Source: CAD feature listing. Evaluate the final solid. Frame: model axes, mm. Face numbers are marked on the shaded views. A direction names the side the tool comes from. Round coordinates to 2 decimals unless told otherwise and drop trailing zeros. Loops run counter-clockwise (first coordinate to the right, second up) from the corner with the lowest first, then second, coordinate; pieces in that order, holes last.
Item 1: Access query for the marked faces 5, 6, 7, 8 and 9. Directions: +Z, -Z, +X, -X, +Y, -Y. A direction counts if a zero-diameter tool reaches every point of the face in a straight line with its end or side. Return the directions, or none.
Item 2: Section query B-B on x = -0.25. Return loops of the section in (y, z), then the cut area to 3 significant figures.
Item 3: Section query A-A on z = 0.4. Return loops of the section in (x, y), then the cut area to 3 significant figures.
Item 4: Pull-direction query (X, two-part tool) for the marked faces 1, 2, 3 and 4; classes: released by +X, released by -X, zero draft, split by the parting line, or undercut.
Item 5: Section query D-D on y = -2.55. Return loops of the section in (x, z).
Item 6: First-contact query: P1, Ø0.8, axis at y = -2.5, z = 1, coming from the -X side; P2, Ø1.1, axis at y = 2.5, z = 1.5, coming from the +X side; P3, Ø3, axis at x = -2, z = 3.5, coming from the -Y side. Flat tips, straight axial feed; report the tip coordinate or a pass-through.
Item 7: Ray query, L1, parallel to Y at x = -3, z = 3.45; L2, parallel to Y at x = -0.5, z = 1.05; L3, parallel to Y at x = 1.75, z = 2.2. Return the intervals inside material, ascending.
Item 8: Section query C-C on x = 1.25. Return loops of the section in (y, z).
```python
from build123d import *

# Parameters (mm, degrees)
BOSS_EXTRUDE1_DEPTH = 6
CUT_EXTRUDE1_DEPTH  = 2
CUT_EXTRUDE2_DEPTH  = 2
CUT_EXTRUDE3_DEPTH  = 2
CUT_EXTRUDE4_DEPTH  = 3


with BuildPart() as part:
    # Sketch1 → Boss-Extrude1 (new body)
    with BuildSketch(Plane.XY):
        with BuildLine():
            Line((0, 2), (-4, 2))
            Line((-4, 2), (-4, 3))
            Line((-4, 3), (0, 3))
            ThreePointArc((0, 3), (3, 0), (0, -3))
            Line((0, -3), (-1, -3))
            Line((-1, -3), (-1, -2))
            Line((-1, -2), (0, -2))
            ThreePointArc((0, -2), (2, 0), (0, 2))
        make_face()
    extrude(amount=BOSS_EXTRUDE1_DEPTH)

    # Sketch2 → Cut-Extrude1 (cut)
    with BuildSketch(Plane.XY.offset(6)):
        with BuildLine():
            Line((3, 0), (2, 0))
            ThreePointArc((2, 0), (1.414213562, -1.414213562), (0, -2))
            Line((0, -2), (0, -3))
            ThreePointArc((0, -3), (2.121320344, -2.121320344), (3, 0))
        make_face()
    extrude(amount=-CUT_EXTRUDE1_DEPTH, mode=Mode.SUBTRACT)

    # Sketch3 → Cut-Extrude2 (cut)
    with BuildSketch(Plane.XZ.offset(3)):
        Polygon((0, 4), (-1, 2), (-1, 6), (0, 6), align=None)
    extrude(amount=-CUT_EXTRUDE2_DEPTH, mode=Mode.SUBTRACT)

    # Sketch4 → Cut-Extrude3 (cut)
    with BuildSketch(Plane.XZ.offset(-2)):
        with BuildLine():
            Line((-1, 5), (0, 5))
            Line((0, 5), (0, 6))
            Line((0, 6), (-4, 6))
            Line((-4, 6), (-4, 2))
            ThreePointArc((-4, 2), (-3.121320344, 4.121320344), (-1, 5))
        make_face()
    extrude(amount=-CUT_EXTRUDE3_DEPTH, mode=Mode.SUBTRACT)

    # Sketch5 → Cut-Extrude4 (cut)
    with BuildSketch(Plane(origin=(0, 3, 0), x_dir=(1, 0, 0), z_dir=(0, 1, 0))):
        with BuildLine():
            Line((-2, 0), (-2, -2))
            ThreePointArc((-2, -2), (-1, -3), (0, -2))
            Line((0, -2), (0, 0))
            Line((0, 0), (-2, 0))
        make_face()
    extrude(amount=-CUT_EXTRUDE4_DEPTH, mode=Mode.SUBTRACT)


solid = part.part
```
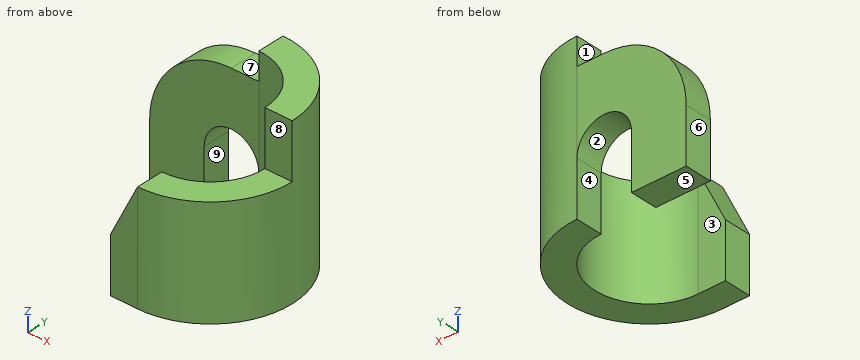
Data:
1. face 5: -Z, +X, -X, +Y, -Y
1. face 6: +Z, -Z, -X, +Y, -Y
1. face 7: +Z, -X, +Y, -Y
1. face 8: +Z, +X, -X, -Y
1. face 9: -Z, +Y, -Y
2. outline: (-3, 0) - (-2, 0) - (-2, 3.5) - (-3, 3.5) - close; (2, 2.66) - (3, 2.66) - (3, 5) - (2, 5) - close
2. area: 5.84 mm2
3. outline: (-4, 2) - (-2, 2) - (-2, 3) - (-4, 3) - close; (-1, -3) - (0, -3) arc R3 ccw to (0, 3) - (0, 2) arc R2 cw to (0, -2) - (-1, -2) - close
3. area: 10.9 mm2
4. face 1: released by -X
4. face 2: undercut
4. face 3: zero draft
4. face 4: undercut
5. outline: (-1, 0) - (1.58, 0) - (1.58, 4) - (0, 4) - (-1, 2) - close
6. P1: stops at x = -1
6. P2: stops at x = 2.28
6. P3: stops at y = 2
7. L1: y = 2 to 3
7. L2: y = -3 to -2
7. L3: y = -2.44 to -0.97, 0.97 to 2.44
8. outline: (-2.73, 0) - (-1.56, 0) - (-1.56, 4) - (-2.73, 4) - close; (1.56, 0) - (2.73, 0) - (2.73, 6) - (1.56, 6) - close
